CAD build for the part. Positions are in the model's coordinates, mm. Face numbers are marked on the shaded views. A direction names the side the tool comes from. Give positions to 0.01 mm unless a question says otherwise; leave off trailing zeros. Write each loop counter-clockwise with the first axis right and the second up, starting at its lowest first coordinate (ties: lowest second). Pieces come first, ordered by that corner, then holes. Notation, with made-up numbers: (-1.75, 12) -> (25.25, 12) arc R21 cw to (25.25, 31) -> close; hole circle Ø7 at (64.5, 59.5). An arc over 180 degrees is marked (long way). Answer as a JSON object with one key per item and string values.
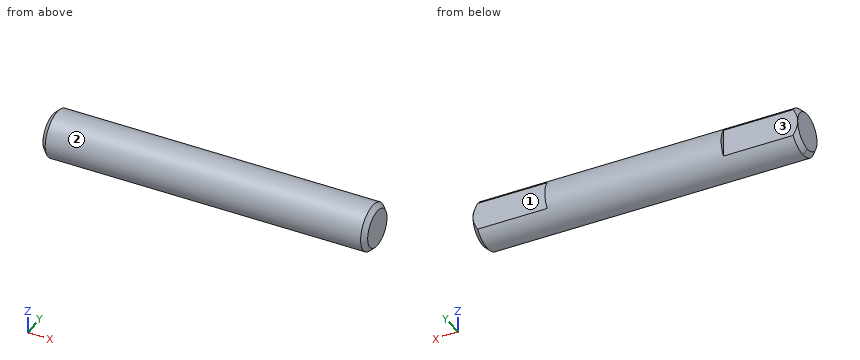
```python
from build123d import *

# Parameters (mm, degrees)
SKETCH1_R           = 2.5
BOSS_EXTRUDE1_DEPTH = 17.5
SKETCH2_W           = 7.702473448
SKETCH2_H           = 1.959232648
CUT_EXTRUDE1_DEPTH  = 28.230497608
CHAMFER4_SIZE       = 0.5
CHAMFER5_SIZE       = 0.5


with BuildPart() as part:
    # Sketch1 → Boss-Extrude1 (new, symmetric)
    with BuildSketch(Plane(origin=(0, 0, 0), x_dir=(0, 0, -1), z_dir=(1, 0, 0))):
        Circle(SKETCH1_R)
    extrude(amount=BOSS_EXTRUDE1_DEPTH, both=True)

    # Sketch2 → Cut-Extrude1 (cut, through all)
    with BuildSketch(Plane(origin=(9.5, 0, 0), x_dir=(0, 0, -1), z_dir=(1, 0, 0))):
        with Locations((0.148863265, 2.979616324)):
            Rectangle(SKETCH2_W, SKETCH2_H)
    cut_extrude1 = extrude(amount=CUT_EXTRUDE1_DEPTH, mode=Mode.SUBTRACT)

    # Mirror1: Cut-Extrude1 across plane
    add(cut_extrude1.mirror(Plane(origin=(0, 0, 0), x_dir=(0, 0, 1), z_dir=(1, 0, 0))), mode=Mode.SUBTRACT)

    # Chamfer4
    chamfer4_edges = [part.edges().sort_by_distance(p)[0] for p in [
        (17.5, -2.236067977, 1.118033989),
    ]]
    chamfer(chamfer4_edges, length=CHAMFER4_SIZE - 0.0001)  # a hair under: the kernel refuses the full size

    # Chamfer5
    chamfer5_edges = [part.edges().sort_by_distance(p)[0] for p in [
        (-17.5, -2.236067977, 1.118033989),
    ]]
    chamfer(chamfer5_edges, length=CHAMFER5_SIZE - 0.0001)  # a hair under: the kernel refuses the full size


solid = part.part
```
1) Wall check: probe 1 along X at (y, z) = (-2, 0.1); probe 2 along Y at (x, z) = (-3, 0.1); probe 3 along Y at (x, z) = (11.5, -0.6). Give the ranges that are in metal, low to high.
Model answer:
{"probe 1": "x = -17.5 to 17.5", "probe 2": "y = -2.5 to 2.5", "probe 3": "y = -2.43 to 2"}
2) 3-axis set-ups, long thin cutter, end or side, ignore diameter. For the marked faces 1, 2 and 3: which of +Z, -Z, +X, -X, +Y, -Y reach the whole face in a straight line?
Model answer:
{"face 1": "+Z, -Z, +X, +Y", "face 2": "+X, -X", "face 3": "+Z, -Z, -X, +Y"}
3) Slice it at A-A (x = 7). List the corners of the cut face in (y, z), then the cut area to 3 significant figures.
Model answer:
{"outline": "circle Ø5 at (0, 0)", "area": "19.6 mm2"}
4) Slice it at B-B (x = 13). List the corners of the cut face in (y, z).
Model answer:
{"outline": "(2, -1.5) -> (2, 1.5) arc R2.5 ccw (long way) to start"}
5) Pin check, flat tips, straight feed: pin 1 (2 mm diameter, centred on x = -10, z = 1.5, fed in from -Y); pin 2 (0.6 mm diameter, centred on y = 2.5, z = -0.5, fed in from -X); pin 3 (1.5 mm diameter, centred on x = 13, z = 0.5, fed in from +Y). Stop position of each tip, or through.
Model answer:
{"pin 1": "stops at y = -2.45", "pin 2": "stops at x = -9.5", "pin 3": "stops at y = 2"}
